The listing builds one solid part. Answer for the finished solid, in the listing's coordinates (mm). A direction names the side the tool comes from. Round coordinates to 2 decimals unless told otherwise and drop trailing zeros. Write each loop counter-clockwise with the first axis right and the second up, starting at its lowest first coordinate (ties: lowest second). Pieces come first, ordered by that corner, then holes. Notation, with made-up numbers: (-30, 56) - (12, 56) arc R11 ccw to (12, 65) - close; hole circle Ø4 at (4.25, 64). An arc over 180 degrees is marked (long way). Return JSON: item names as keys, results as strings. Group by question number.
(1) Which of the six approach directions +Z, -Z, +X, -X, +Y, -Y give full straight-line access (tool end or side, diameter ignored) to faces 4 (the flat face through (3, 248.9, -3)), 5 (the flat face through (3, 282.7, -132)), 6 (the flat face through (3, 64.75, -13)), 7 (the flat face through (3, 24.1, -3))?
(2) Section A-A, the plane y = 27.9 is taken. Write down the section's boundary in (x, z), then the cut area to 3 significant figures.
(3) Section C-C, the plane x = 2.6 is taken. Give the number of separate pieces and of enclosed holes in the cut face, then the cut area to 3 significant figures.
(4) Find the intervals of material crossed by line 1 along Z through (x, y) = (2.95, 59.8); line 2 along Y through (x, z) = (2.1, -93.5); line 3 along Y through (x, z) = (2.05, -61), in increasing order. Write a range as [from, to].
(5) Section D-D, the plane y = 254 is taken. Write down the section's boundary in (x, z), then the cut area to 3 significant figures.
(6) Section B-B, the plane z = -40 is taken. Write down the section's boundary in (x, y), then the cut area to 3 significant figures.
(7) Each of these flat-tipped pins is pushed along its axis until it touches: pin 1 (1.8 mm diameter, centred on x = 3.5, y = 137.5, fed in from +Z); pin 2 (3 mm diameter, centred on x = 3.5, z = -11.5, fed in from +Y); pin 3 (2 mm diameter, centred on y = 175.5, z = -27, fed in from -X); pin 4 (3 mm diameter, centred on x = 3.5, z = -2, fed in from -Y). Where does it stop, or does it pass through?
(8) Determine the mould class of faces 1 (the flat face through (3, 63.25, -13)), 2 (the flat face through (3, 286, -177.2)), 3 (the flat face through (3, 269, -181)) for opening direction Z: +Z half, -Z half, draft (parallel to the pull), parting line (faces both ways), or undercut.
```python
from build123d import *

# Parameters (mm, degrees)
ESBO_O1_W                  = 6
ESBO_O1_H                  = 29.8
RESSALTO_EXTRUS_O3_DEPTH   = 187
RESSALTO_EXTRUS_O3_2_DEPTH = 187
RESSALTO_EXTRUS_O3_3_DEPTH = 187
RESSALTO_EXTRUS_O3_4_DEPTH = 187
ESBO_O2_W                  = 175
ESBO_O2_H                  = 289.8
RESSALTO_EXTRUS_O4_DEPTH   = 6
ESBO_O3_W                  = 15
ESBO_O3_H                  = 1.5
CORTE_EXTRUS_O1_DEPTH      = 6
ESBO_O5_R                  = 1.75
ESBO_O5_W                  = 30
ESBO_O5_H                  = 6.2
CORTE_EXTRUS_O3_DEPTH      = 22.8
ESBO_O6_W                  = 20.4
ESBO_O6_H                  = 6.2
CORTE_EXTRUS_O4_DEPTH      = 14.6
FILETE1_R                  = 0.75
CORTE_EXTRUS_O5_DEPTH      = 10
ESBO_O8_R                  = 6.1
CORTE_EXTRUS_O6_DEPTH      = 22


with BuildPart() as part:
    # Esbo_o1 → Ressalto-extrus_o3 (new body)
    with BuildSketch(Plane.XY):
        with Locations((3, 39)):
            Rectangle(ESBO_O1_W, ESBO_O1_H)
    extrude(amount=-RESSALTO_EXTRUS_O3_DEPTH)



with BuildPart() as body_2:
    # Esbo_o1 → Ressalto-extrus_o3 2 (new body)
    with BuildSketch(Plane.XY):
        with Locations((3, 89)):
            Rectangle(ESBO_O1_W, ESBO_O1_H)
    extrude(amount=-RESSALTO_EXTRUS_O3_2_DEPTH)


with BuildPart() as body_3:
    # Esbo_o1 → Ressalto-extrus_o3 3 (new body)
    with BuildSketch(Plane.XY):
        with Locations((3, 184)):
            Rectangle(ESBO_O1_W, ESBO_O1_H)
    extrude(amount=-RESSALTO_EXTRUS_O3_3_DEPTH)


with BuildPart() as body_4:
    # Esbo_o1 → Ressalto-extrus_o3 4 (new body)
    with BuildSketch(Plane.XY):
        with Locations((3, 234)):
            Rectangle(ESBO_O1_W, ESBO_O1_H)
    extrude(amount=-RESSALTO_EXTRUS_O3_4_DEPTH)


with BuildPart() as part_1:
    add(part.part)

    add(body_2.part)  # Ressalto-extrus_o4 merges body 2

    add(body_3.part)  # Ressalto-extrus_o4 merges body 3

    add(body_4.part)  # Ressalto-extrus_o4 merges body 4
    # Esbo_o2 → Ressalto-extrus_o4 (add)
    with BuildSketch(Plane.ZY):
        with Locations((-93.5, 144)):
            Rectangle(ESBO_O2_W, ESBO_O2_H)
    extrude(amount=-RESSALTO_EXTRUS_O4_DEPTH)

    # Esbo_o3 → Corte-extrus_o1 (cut)
    with BuildSketch(Plane.ZY):
        with Locations((-173.5, 64)):
            Rectangle(ESBO_O3_W, ESBO_O3_H)
        with Locations((-13.5, 64)):
            Rectangle(ESBO_O3_W, ESBO_O3_H)
        with Locations((-13.5, 209)):
            Rectangle(ESBO_O3_W, ESBO_O3_H)
        with Locations((-173.5, 209)):
            Rectangle(ESBO_O3_W, ESBO_O3_H)
    extrude(amount=-CORTE_EXTRUS_O1_DEPTH, mode=Mode.SUBTRACT)

    # Esbo_o5 → Corte-extrus_o3 (cut)
    with BuildSketch(Plane.ZY):
        with Locations(Location((-93.5, 59.8, 0), (0, 0, 270))):
            Circle(ESBO_O5_R)
        with Locations((-136, 59.8)):
            Rectangle(ESBO_O5_W, ESBO_O5_H)
        with Locations((-51, 59.8)):
            Rectangle(ESBO_O5_W, ESBO_O5_H)
    extrude(amount=-CORTE_EXTRUS_O3_DEPTH, mode=Mode.SUBTRACT)

    # Esbo_o6 → Corte-extrus_o4 (cut)
    with BuildSketch(Plane.ZY):
        with Locations((-20, 285.8)):
            Rectangle(ESBO_O6_W, ESBO_O6_H)
        with Locations((-55, 285.8)):
            Rectangle(ESBO_O6_W, ESBO_O6_H)
    corte_extrus_o4 = extrude(amount=-CORTE_EXTRUS_O4_DEPTH, mode=Mode.SUBTRACT)

    # Espelhar1: Corte-extrus_o4 across plane
    add(corte_extrus_o4.mirror(Plane.XY.offset(-93.5)), mode=Mode.SUBTRACT)

    # Filete1
    filete1_edges = [part_1.edges().sort_by_distance(p)[0] for p in [
        (3, 64.75, -166),
        (3, 63.25, -166),
        (3, 63.25, -21),
        (3, 64.75, -21),
        (3, 208.25, -21),
        (3, 209.75, -21),
        (3, 208.25, -166),
        (3, 209.75, -166),
    ]]
    fillet(filete1_edges, radius=FILETE1_R - 0.0001)  # a hair under: the kernel refuses the full size

    # Esbo_o7 → Corte-extrus_o5 (cut)
    with BuildSketch(Plane.ZY):
        with BuildLine():
            ThreePointArc((-91.75, 285.8), (-93.404579917, 287.547396637), (-95.239594295, 285.990556265))
            Line((-95.239594295, 285.990556265), (-91.760405705, 285.609443735))
            ThreePointArc((-91.760405705, 285.609443735), (-91.752603363, 285.704579917), (-91.75, 285.8))
        make_face()
        with BuildLine():
            Line((-91.760405705, 285.609443735), (-95.239594295, 285.990556265))
            ThreePointArc((-95.239594295, 285.990556265), (-93.690556265, 284.060405705), (-91.760405705, 285.609443735))
        make_face()
    extrude(amount=-CORTE_EXTRUS_O5_DEPTH, mode=Mode.SUBTRACT)

    # Esbo_o8 → Corte-extrus_o6 (cut)
    with BuildSketch(Plane.ZY):
        with Locations(Location((-29.9, 27.9, 0), (0, 0, 270))):
            Circle(ESBO_O8_R)
    extrude(amount=-CORTE_EXTRUS_O6_DEPTH, mode=Mode.SUBTRACT)


solid = part_1.part
```
Working result:
{
 "1": {"face 4": "+Z, +X, -X, +Y", "face 5": "+X, -X, +Y", "face 6": "+Z, +X, -X", "face 7": "+Z, +X, -X, -Y"},
 "2": {"outline": "(0, -187) - (6, -187) - (6, -36) - (0, -36) - close; (0, -23.8) - (6, -23.8) - (6, 0) - (0, 0) - close", "area": "1,050 mm^2"},
 "3": {"separate pieces": "1", "enclosed holes": "5", "area": "51,000 mm^2"},
 "4": {"line 1": "z = [-181, -151], [-121, -95.25], [-91.75, -66], [-36, -6]", "line 2": "y = [-0.9, 58.05], [61.55, 284.05], [287.55, 288.9]", "line 3": "y = [-0.9, 56.7], [62.9, 282.7]"},
 "5": {"outline": "(0, -181) - (6, -181) - (6, -6) - (0, -6) - close", "area": "1,050 mm^2"},
 "6": {"outline": "(0, -0.9) - (6, -0.9) - (6, 56.7) - (0, 56.7) - close; (0, 62.9) - (6, 62.9) - (6, 288.9) - (0, 288.9) - close", "area": "1,700 mm^2"},
 "7": {"pin 1": "stops at z = -6", "pin 2": "stops at y = 282.7", "pin 3": "stops at x = 0", "pin 4": "stops at y = 24.1"},
 "8": {"face 1": "draft", "face 2": "undercut", "face 3": "-Z half"}
}
